Source: CAD feature listing. Evaluate the final solid. Frame: model axes, mm. A direction names the side the tool comes from. Round coordinates to 2 decimals unless told otherwise and drop trailing zeros. Order: outer loops, then holes, each group sorted by start corner. A loop starts at its lowest first (then second) coordinate and runs counter-clockwise, first axis right, second up. Notation, with made-up numbers: M -30.5,-38 L 8.5,-38 A27 cw 8.5,-6 Z; hole C 3,4 d7. An arc over 180 degrees is marked long. Answer as CSV lines item,"result". Start each with the question number.
Item 1: Section query D-D on z = 2.25. Return the cut outline in (x, y), plus the area to 3 significant figures.
Item 2: First-contact query: P1, Ø1.5, axis at x = -8, z = 13.5, coming from the +Y side; P2, Ø2, axis at x = -9.5, z = 5, coming from the -Y side; P3, Ø1, axis at x = -4, z = 11.5, coming from the +Y side. Flat tips, straight axial feed; report the tip coordinate or a pass-through.
Item 3: Set-up query: faces 1 (the face through (-4.56, 0.09, 0.52)), 2 (the face through (0, 3.25, 7)), 3 (the face through (4.56, 0.09, 14.48)). Return all of +Z, -Z, +X, -X, +Y, -Y with unobstructed straight access to the full face (end or side cutting, diameter ignored); none if empty.
Item 4: Pull-direction query (X, two-part tool) for faces 4 (the face through (8, 0, 15)), 5 (the face through (0.09, 4.56, 14.48)), 6 (the face through (-13.887, -10.648, 7.479)); classes: +X half, -X half, draft (parallel to the pull), parting line (faces both ways), or undercut.
Item 5: Line query: line 1 (X direction, y = 2, z = 9); line 2 (X direction, y = 1.5, z = 13.25); line 3 (Z direction, x = 6, y = 5.5). Output: solid intervals per line, ascending. Write a range as [from, to].
Item 6: Section query C-C on z = 6.5. Return the cut outline in (x, y).
Item 7: Section query A-A on y = 0. Return the cut outline in (x, z), plus the area to 3 significant figures.
from build123d import *

# Parameters (mm, degrees)
F0_R     = 17.5
F0_W     = 6.5
F0_H     = 6.5
F1_DEPTH = 15
F2_R     = 6
F3_R     = 3


# Not quite as in the source:
# - a feature names something its author has since deleted; it is built from what else it names


with BuildPart() as f1:
    # F0 (on Top) → F1 (new body)
    with BuildSketch(Plane.XY):
        Circle(F0_R)
        Rectangle(F0_W, F0_H, mode=Mode.SUBTRACT)
    extrude(amount=F1_DEPTH)

    # F2
    f2_edges = [f1.edges().sort_by_distance(p)[0] for p in [
        (-17.5, 0, 15),
        (-17.5, 0, 0),
    ]]
    fillet(f2_edges, radius=F2_R)

    # F3
    f3_edges = [f1.edges().sort_by_distance(p)[0] for p in [
        (-3.25, 0, 15),
        (0, 3.25, 15),
        (3.25, 0, 15),
        (0, -3.25, 15),
        (0, 3.25, 0),
        (-3.25, 0, 0),
        (0, -3.25, 0),
        (3.25, 0, 0),
    ]]
    fillet(f3_edges, radius=F3_R)


solid = f1.part
Results:
1,outline,"C 0,0 d32.37; hole M -3.35,-3.35 L 3.35,-3.35 L 3.35,3.35 L -3.35,3.35 Z"
1,area,"778 mm^2"
2,P1,"y = 14.18"
2,P2,"y = -15.23"
2,P3,"y = 16.72"
3,face 1,"-Z"
3,face 2,"+Z, -Z"
3,face 3,"+Z"
4,face 4,"draft"
4,face 5,"undercut"
4,face 6,"parting line"
5,line 1,"[-17.39, -3.25], [3.25, 17.39]"
5,line 2,"[-15.66, -3.52], [3.52, 15.66]"
5,line 3,"[0.01, 14.99]"
6,outline,"C 0,0 d35; hole M -3.25,-3.25 L 3.25,-3.25 L 3.25,3.25 L -3.25,3.25 Z"
7,outline,"M -17.5,6 A6 ccw -11.5,0 L -6.25,0 A3 ccw -3.25,3 L -3.25,12 A3 ccw -6.25,15 L -11.5,15 A6 ccw -17.5,9 Z; M 3.25,3 A3 ccw 6.25,0 L 11.5,0 A6 ccw 17.5,6 L 17.5,9 A6 ccw 11.5,15 L 6.25,15 A3 ccw 3.25,12 Z"
7,area,"389 mm^2"
